from build123d import *

# Parameters (mm, degrees)
F0_DEPTH = 2
F1_W     = 5
F1_H     = 2
F2_DEPTH = 25


# Not quite as in the source:
# - a feature names something its author has since deleted; it is built from what else it names


with BuildPart() as f0:
    # F3 (on Top) → F0 (new body)
    with BuildSketch(Plane.XY):
        Polygon((-40, 0), (-2, 0), (-2, 40), (-40, 40), (-40, 32), (-42, 32), (-42, 24), (-40, 24), (-40, 16), (-42, 16), (-42, 8), (-40, 8), align=None)
    extrude(amount=F0_DEPTH)

    # F1 (on Top) → F2 (cut)
    with BuildSketch(Plane.XY):
        with Locations((-29.5, 16)):
            Rectangle(F1_W, F1_H)
    extrude(amount=F2_DEPTH, mode=Mode.SUBTRACT)


solid = f0.part
Model file for the job. Use its own axes, mm. A direction names the side the tool comes from. Give positions to 0.01 mm unless a question says otherwise; leave off trailing zeros. Order: outer loops, then holes, each group sorted by start corner. A loop starts at its lowest first (then second) coordinate and runs counter-clockwise, first axis right, second up. Notation, with made-up numbers: M 49,-33 L 84,-33 A24 cw 84,-13 Z; hole C 5.25,37 d6. An arc over 180 degrees is marked long. Write item = value, one per line.
Q1. Cut at B-B, the plane z = 1.1. List the corners of the cut face in (x, y).
Derived:
outline = M -42,8 L -40,8 L -40,0 L -2,0 L -2,40 L -40,40 L -40,32 L -42,32 L -42,24 L -40,24 L -40,16 L -42,16 Z; hole M -32,15 L -27,15 L -27,17 L -32,17 Z
Q2. Cut at A-A, the plane x = -30. List the corners of the cut face in (y, z), then the cut area to 3 significant figures.
Derived:
outline = M 0,0 L 15,0 L 15,2 L 0,2 Z; M 17,0 L 40,0 L 40,2 L 17,2 Z
area = 76.0 mm2
Q3. Tool access for faces 1 (the flat face through (-40, 20, 1)), 2 (the flat face through (-41, 8, 1)), 3 (the flat face through (-40, 36, 1)), 4 (the flat face through (-30, 15, 1)): list every direction of +Z, -Z, +X, -X, +Y, -Y with a clear straight run to the whole face (end or side of a thin tool).
Derived:
face_1 = +Z, -Z, -X
face_2 = +Z, -Z, -X, -Y
face_3 = +Z, -Z, -X, +Y
face_4 = +Z, -Z
Q4. Drill centre lines: line 1 (Y direction, x = -28, z = 1.2); line 2 (X direction, y = 36, z = 0.75). Where is each one in solid material? Low to high. Write a range as [from, to].
Derived:
line_1 = [0, 15], [17, 40]
line_2 = [-40, -2]
Q5. Cut at C-C, the plane y = 4.5. List the corners of the cut face in (x, z).
Derived:
outline = M -40,0 L -2,0 L -2,2 L -40,2 Z
Q6. Flat gauge pins, fed straight in: pin 1 (0.6 mm diameter, centred on x = -41, z = 1, fed in from -Y); pin 2 (1 mm diameter, centred on y = 38, z = 1, fed in from -X); pin 3 (1 mm diameter, centred on x = -41.5, z = 0.5, fed in from +Y). Where does each tip first touch, or does it go through?
Derived:
pin_1 = 8
pin_2 = -40
pin_3 = 32
Q7. Two-plate mould, pull along Y, no slides. Class faces 5 (the flat face through (-21, 0, 1)), 6 (the flat face through (-41, 16, 1)), 7 (the flat face through (-21, 40, 1)), 8 (the flat face through (-40, 4, 1)): pulls with the +Y half, pulls with the -Y half, needs draft (parallel to the pull), parting line crosses it, or undercut.
Derived:
face_5 = pulls with the -Y half
face_6 = undercut
face_7 = pulls with the +Y half
face_8 = needs draft
